```python
from build123d import *

# Parameters (mm, degrees)
SKETCH1_R           = 2.5
SKETCH1_R_2         = 1.45
BOSS_EXTRUDE1_DEPTH = 1.5
SKETCH2_W           = 47.7875
SKETCH2_H           = 2
CUT_EXTRUDE1_DEPTH  = 2.5


with BuildPart() as part:
    # Sketch1 → Boss-Extrude1 (new body)
    with BuildSketch(Plane.XY):
        with BuildLine():
            Line((24.2875, 244.4875), (24.2875, 200.7375))
            ThreePointArc((24.2875, 200.7375), (22.823033906, 197.201966094), (19.2875, 195.7375))
            Line((19.2875, 195.7375), (10, 195.7375))
            ThreePointArc((10, 195.7375), (2.928932188, 192.808567812), (0, 185.7375))
            Line((0, 185.7375), (0, 11))
            Line((0, 11), (-5, 11))
            Line((-5, 11), (-5, 0))
            Line((-5, 0), (0, 0))
            Line((0, 0), (0, -11))
            Line((0, -11), (155.575, -11))
            Line((155.575, -11), (155.575, 0))
            Line((155.575, 0), (160.575, 0))
            Line((160.575, 0), (160.575, 11))
            Line((160.575, 11), (155.575, 11))
            Line((155.575, 11), (155.575, 50.954595736))
            ThreePointArc((155.575, 50.954595736), (152.164764791, 58.476231197), (144.26, 60.867757442))
            ThreePointArc((144.26, 60.867757442), (127.2875, 75.7375), (144.26, 90.607242558))
            ThreePointArc((144.26, 90.607242558), (152.164764791, 92.998768803), (155.575, 100.520404264))
            Line((155.575, 100.520404264), (155.575, 185.7375))
            ThreePointArc((155.575, 185.7375), (152.646067812, 192.808567812), (145.575, 195.7375))
            Line((145.575, 195.7375), (128.6625, 195.7375))
            ThreePointArc((128.6625, 195.7375), (118.055898282, 200.130898282), (113.6625, 210.7375))
            Line((113.6625, 210.7375), (113.6625, 244.4875))
            ThreePointArc((113.6625, 244.4875), (112.198033906, 248.023033906), (108.6625, 249.4875))
            Line((108.6625, 249.4875), (29.2875, 249.4875))
            ThreePointArc((29.2875, 249.4875), (25.751966094, 248.023033906), (24.2875, 244.4875))
        make_face()
        with Locations((14.2875, 185.7375)):
            Circle(SKETCH1_R, mode=Mode.SUBTRACT)
        with Locations((141.2875, 185.7375)):
            Circle(SKETCH1_R, mode=Mode.SUBTRACT)
        with Locations((108.6625, 212.7375)):
            Circle(SKETCH1_R_2, mode=Mode.SUBTRACT)
        with Locations((108.6625, 244.4875)):
            Circle(SKETCH1_R_2, mode=Mode.SUBTRACT)
        with Locations((29.2875, 244.4875)):
            Circle(SKETCH1_R_2, mode=Mode.SUBTRACT)
        with Locations((29.2875, 212.7375)):
            Circle(SKETCH1_R_2, mode=Mode.SUBTRACT)
        with Locations((132.2875, 167.7375)):
            Circle(SKETCH1_R, mode=Mode.SUBTRACT)
        with Locations((92.2875, 207.7375)):
            Circle(SKETCH1_R, mode=Mode.SUBTRACT)
    extrude(amount=BOSS_EXTRUDE1_DEPTH)

    # Sketch2 → Cut-Extrude1 (cut, through all)
    with BuildSketch(Plane.XY.offset(1.5)):
        with Locations((38.89375, -1)):
            Rectangle(SKETCH2_W, SKETCH2_H)
        with Locations((116.68125, -1)):
            Rectangle(SKETCH2_W, SKETCH2_H)
    extrude(amount=-CUT_EXTRUDE1_DEPTH, mode=Mode.SUBTRACT)


solid = part.part
```
The model under review builds one solid part; all positions refer to its coordinate system, in mm. Give positions to 0.01 mm unless a question says otherwise; leave off trailing zeros. Loops run counter-clockwise (first coordinate to the right, second up) from the corner with the lowest first, then second, coordinate; pieces in that order, holes last. Notation, with made-up numbers: (56.5, -10) -> (88.5, -10) arc R9 cw to (88.5, 4) -> close; hole circle Ø3 at (-35.75, -33). An arc over 180 degrees is marked (long way). Use CSV: the item, a comma, the result in double quotes.
1. Consider section D-D, the plane y = 232.5. Write out the cut boundary in (x, z), then the cut area to 3 significant figures.
Result:
outline,"(24.29, 0) -> (113.66, 0) -> (113.66, 1.5) -> (24.29, 1.5) -> close"
area,"134 mm²"
2. Consider section B-B, the plane y = 134.5. Write out the cut boundary in (x, z) (3 decimals), then the cut area to 3 significant figures.
Result:
outline,"(0, 0) -> (155.575, 0) -> (155.575, 1.5) -> (0, 1.5) -> close"
area,"233 mm²"
3. The part is to be moulded in two halves that separate along X. For faces 1 (the face through (25.79, 248.06, 0.74)), 2 (the face through (15.4, 183.5, 0.7)), 3 (the face through (77, 121, 1.5)), say which applies: +X half, -X half, draft (parallel to the pull), parting line (faces both ways), or undercut.
Result:
face 1,"-X half"
face 2,"undercut"
face 3,"draft"
4. For P1, Ø6.5, axis at x = 132.29, y = 167.74, coming from the -Z side; P2, Ø0.8, axis at y = -0.5, z = 1, coming from the +X side (3 decimals); P3, Ø0.8, axis at y = 220.5, z = 0.5, coming from the +X side, all flat-tipped, find the tip position at first contact; note any pin that passes through.
Result:
P1,"stops at z = 0"
P2,"stops at x = 155.575"
P3,"stops at x = 113.66"
5. To check wall thickness, follow probe 1 along Y at (x, z) = (107, 1.45); probe 2 along Y at (x, z) = (142, 0.75); probe 3 along X at (y, z) = (43, 1.45) (3 decimals). State the ranges of each line that lie inside material, in increasing order. Write a range as from..to.
Result:
probe 1,"y = -11..-2, 0..249.49"
probe 2,"y = -11..60.74, 90.73..183.34, 188.13..195.74"
probe 3,"x = 0..155.575"
6. Consider section C-C, the plane z = 0.8. Count the separate pieces of the cut face and the enclosed holes in it, then the cut area to 3 significant figures.
Result:
separate pieces,"1"
enclosed holes,"10"
area,"36,000 mm²"
7. Consider section A-A, the plane x = 123. Write out the cut boundary in (y, z), then the cut area to 3 significant figures.
Result:
outline,"(-11, 0) -> (-2, 0) -> (-2, 1.5) -> (-11, 1.5) -> close; (0, 0) -> (196.85, 0) -> (196.85, 1.5) -> (0, 1.5) -> close"
area,"309 mm²"
